Part model, mm, in its own coordinate system. A direction names the side the tool comes from. Give positions to 0.01 mm unless a question says otherwise; leave off trailing zeros. Loops run counter-clockwise (first coordinate to the right, second up) from the corner with the lowest first, then second, coordinate; pieces in that order, holes last. Notation, with made-up numbers: (72.25, -19) -> (89.25, -19) arc R18 cw to (89.25, -9) -> close; hole circle Ø6 at (-5, 4). An arc over 180 degrees is marked (long way). Write item = value, one per line.
from build123d import *

# Parameters (mm, degrees)
SKETCH1_W           = 5
SKETCH1_H           = 15.35
BOSS_EXTRUDE1_DEPTH = 24
SKETCH2_R           = 1.5
CUT_EXTRUDE1_DEPTH  = 77.425192182
CUT_EXTRUDE4_REACH  = 50.199
SKETCH8_W           = 22.75
SKETCH8_H           = 12
SKETCH9_R           = 0.75
CUT_EXTRUDE5_DEPTH  = 49.198781105


with BuildPart() as part:
    # Sketch1 → Boss-Extrude1 (new body)
    with BuildSketch(Plane(origin=(0, 0, 0), x_dir=(1, 0, 0), z_dir=(0, 1, 0))):
        with Locations((-32.5, -11.425)):
            Rectangle(SKETCH1_W, SKETCH1_H)
        Polygon((-35, -3.75), (-30, -3.75), (0, -3.75), (0, 3.75), (-35, 3.75), align=None)
        Polygon((0, 3.75), (0, -3.75), (30, -3.75), (35, -3.75), (35, 3.75), align=None)
        with Locations((32.5, -11.425)):
            Rectangle(SKETCH1_W, SKETCH1_H)
    extrude(amount=BOSS_EXTRUDE1_DEPTH)

    # Sketch2 → Cut-Extrude1 (cut, through all)
    with BuildSketch(Plane.ZY.offset(35)):
        with Locations((14.1, 18)):
            Circle(SKETCH2_R)
        with Locations((14.1, 6)):
            Circle(SKETCH2_R)
    extrude(amount=-CUT_EXTRUDE1_DEPTH, mode=Mode.SUBTRACT)

    # Sketch8 → Cut-Extrude4 (cut, up to next)
    with BuildSketch(Plane(origin=(0, 0, -3.75), x_dir=(-1, 0, 0), z_dir=(0, 0, -1)), mode=Mode.PRIVATE) as cut_extrude4_sk1:
        with Locations((-4.875, 12)):
            Rectangle(SKETCH8_W, SKETCH8_H)
    cut_extrude4_tool1 = extrude(cut_extrude4_sk1.sketch, amount=-CUT_EXTRUDE4_REACH, mode=Mode.PRIVATE) & part.part
    add(cut_extrude4_tool1.solids().sort_by_distance((4.875, 12, -3.75))[0], mode=Mode.SUBTRACT)

    # Sketch9 → Cut-Extrude5 (cut, through all)
    with BuildSketch(Plane(origin=(0, 0, -3.75), x_dir=(-1, 0, 0), z_dir=(0, 0, -1))):
        with Locations((-19.16, 12)):
            Circle(SKETCH9_R)
        with Locations((8.64, 12)):
            Circle(SKETCH9_R)
    extrude(amount=-CUT_EXTRUDE5_DEPTH, mode=Mode.SUBTRACT)


solid = part.part
1) Slice it at A-A, the plane x = 19.16. List the corners of the cut face in (y, z), and give its area (3 significant figures).
Resolved:
outline = (0, -3.75) -> (11.25, -3.75) -> (11.25, 3.75) -> (0, 3.75) -> close; (12.75, -3.75) -> (24, -3.75) -> (24, 3.75) -> (12.75, 3.75) -> close
area = 169 mm²
2) Drop flat-ended pins along their axis: P1, Ø12, axis at x = -1, y = 6.5, coming from the +Z side; P2, Ø2.5, axis at y = 6, z = 14.1, coming from the -X side. Give the stop position or say it passes through.
Resolved:
P1 = 3.75
P2 = through
3) Pull direction Y, two halves, no side cores. Call faces 4 (the face through (5, 18, 0)), 5 (the face through (-30, 12, 12)), 6 (the face through (0, 24, 2)), 7 (the face through (0, 0, 2)): pulls with the +Y half, pulls with the -Y half, needs draft (parallel to the pull), parting line crosses it, or undercut.
Resolved:
face_4 = undercut
face_5 = needs draft
face_6 = pulls with the +Y half
face_7 = pulls with the -Y half
4) Which spindle directions (+Z, -Z, +X, -X, +Y, -Y) get a long thin tool onto all of the face, cutting with end or side? Do faces 1 (the face through (32, 12, 19.1)), 2 (the face through (30, 12, 12)), 3 (the face through (-6.5, 12, 0)). Say none if no direction does.
Resolved:
face_1 = +Z, +X, -X, +Y, -Y
face_2 = +Z, +Y, -Y
face_3 = +Z, -Z
5) Drill centre lines: line 1 along Y through (x, z) = (-32.25, 14.1); line 2 along X through (y, z) = (6, 9.25); line 3 along X through (y, z) = (7.25, -1.25). Where is each one in solid material? Low to high. Write a range as [from, to].
Resolved:
line_1 = [0, 4.5], [7.5, 16.5], [19.5, 24]
line_2 = [-35, -30], [30, 35]
line_3 = [-35, -6.5], [16.25, 35]
6) Slice it at C-C, the plane z = 1.75. List the corners of the cut face in (x, y).
Resolved:
outline = (-35, 0) -> (35, 0) -> (35, 24) -> (-35, 24) -> close; hole circle Ø1.5 at (-8.64, 12); hole (-6.5, 6) -> (16.25, 6) -> (16.25, 18) -> (-6.5, 18) -> close; hole circle Ø1.5 at (19.16, 12)
7) Slice it at B-B, the plane z = 11.5. List the corners of the cut face in (x, y).
Resolved:
outline = (-35, 0) -> (-30, 0) -> (-30, 24) -> (-35, 24) -> close; (30, 0) -> (35, 0) -> (35, 24) -> (30, 24) -> close
8) Slice it at D-D, the plane y = 15.75. List the corners of the cut face in (x, z).
Resolved:
outline = (-35, -3.75) -> (-6.5, -3.75) -> (-6.5, 3.75) -> (-30, 3.75) -> (-30, 19.1) -> (-35, 19.1) -> close; (16.25, -3.75) -> (35, -3.75) -> (35, 19.1) -> (30, 19.1) -> (30, 3.75) -> (16.25, 3.75) -> close
